```python
from build123d import *

# Parameters (mm, degrees)
SKETCH_1_W          = 58.6
SKETCH_1_H          = 38
EXTRUDE_1_DEPTH     = 3
SKETCH_2_W          = 4.15
SKETCH_2_H          = 27.5
CUT_EXTRUDE_1_DEPTH = 36.049821683
SKETCH_3_R          = 0.35
CUT_EXTRUDE_2_DEPTH = 3


with BuildPart() as part:
    # 草图1 → 凸台-拉伸1 (new body)
    with BuildSketch(Plane(origin=(0, 0, 0), x_dir=(1, 0, 0), z_dir=(0, 1, 0))):
        Rectangle(SKETCH_1_W, SKETCH_1_H)
    extrude(amount=EXTRUDE_1_DEPTH)

    # 草图2 → 切除-拉伸1 (cut, through all)
    with BuildSketch(Plane.XZ):
        with Locations((-2.775, 0)):
            Rectangle(SKETCH_2_W, SKETCH_2_H)
    extrude(amount=-CUT_EXTRUDE_1_DEPTH, mode=Mode.SUBTRACT)

    # 草图3 → 切除-拉伸2 (cut)
    with BuildSketch(Plane(origin=(29.3, 0, 0), x_dir=(0, 0, -1), z_dir=(1, 0, 0))):
        with Locations((-11.4, 1.5)):
            Circle(SKETCH_3_R)
        with Locations((11.4, 1.5)):
            Circle(SKETCH_3_R)
    extrude(amount=-CUT_EXTRUDE_2_DEPTH, mode=Mode.SUBTRACT)


solid = part.part
```
Could you check a few things on this model? Use its own coordinates, in mm. A direction names the side the tool comes from. Round coordinates to 2 decimals unless told otherwise and drop trailing zeros. Loops run counter-clockwise (first coordinate to the right, second up) from the corner with the lowest first, then second, coordinate; pieces in that order, holes last.
Q1. On a 3-axis mill with a long thin cutter (end or side, diameter ignored), from which of +Z, -Z, +X, -X, +Y, -Y can I reach the whole of each face in a straight line? I mean faces 5 (the flat face through (-29.3, 1, 0)), 6 (the flat face through (-4.85, 1, 0)). Say none if no direction works.
Q2. I want a section at B-B (z = 1.5). Write out the boundary of the cut face in (x, y).
Q3. Please list where these lines run through material, in increasing order: L1, parallel to X at y = 1.65, z = 3; L2, parallel to Z at x = -4.5, y = 0.6; L3, parallel to Y at x = 28.25, z = -11.4.
Q4. I want a section at A-A (x = -2). Write out the boundary of the cut face in (y, z), and give its area (3 significant figures).
Q5. Thinking about a two-plate mould opening in X: for faces 1 (the flat face through (29.3, 1, 0)), 2 (the flat face through (-0.7, 1, 0)), 3 (the flat face through (0, 1, 19)), 4 (the flat face through (-3, 1, -13.75)), which applies, pulls with the +X half, pulls with the -X half, needs draft (parallel to the pull), parting line crosses it, or undercut?
Answer below:
1. face 5: +Z, -Z, -X, +Y, -Y
1. face 6: +Y, -Y
2. outline: (-29.3, 0) - (-4.85, 0) - (-4.85, 3) - (-29.3, 3) - close; (-0.7, 0) - (29.3, 0) - (29.3, 3) - (-0.7, 3) - close
3. L1: x = -29.3 to -4.85, -0.7 to 29.3
3. L2: z = -19 to -13.75, 13.75 to 19
3. L3: y = 0 to 1.15, 1.85 to 3
4. outline: (0, -19) - (3, -19) - (3, -13.75) - (0, -13.75) - close; (0, 13.75) - (3, 13.75) - (3, 19) - (0, 19) - close
4. area: 31.5 mm2
5. face 1: pulls with the +X half
5. face 2: undercut
5. face 3: needs draft
5. face 4: undercut
